Could you check a few things on this model? Use its own coordinates, in mm. A direction names the side the tool comes from. Give positions to 0.01 mm unless a question says otherwise; leave off trailing zeros. Loops run counter-clockwise (first coordinate to the right, second up) from the corner with the lowest first, then second, coordinate; pieces in that order, holes last. Notation, with made-up numbers: (-11, -17) -> (42, -17) arc R18 ccw to (42, -1) -> close; hole circle Ø2 at (79, 0.5). An arc over 180 degrees is marked (long way). Put each result on its own line as item: value.
```python
from build123d import *

# Parameters (mm, degrees)
F1_DEPTH = 63.5
F0_W     = 25.4
F0_H     = 19.05
F2_DEPTH = 25.4
F3_DEPTH = 7.9375


with BuildPart() as f1:
    # F0 (on Front) → F1 (new body, symmetric)
    with BuildSketch(Plane.XZ):
        Polygon((41.275, -9.525), (41.275, 9.525), (22.225, 9.525), (-41.275, 9.525), (-41.275, -9.525), align=None)
    extrude(amount=F1_DEPTH, both=True)

    # F0 (on Front) → F2 (join, symmetric)
    with BuildSketch(Plane.XZ):
        with BuildLine():
            Line((22.225, 9.525), (41.275, 9.525))
            Line((41.275, 9.525), (41.275, 27.0002))
            ThreePointArc((41.275, 27.0002), (45.9246798487, 38.2255201513), (57.15, 42.8752))
            Line((57.15, 42.8752), (60.325, 42.8752))
            Line((60.325, 42.8752), (60.325, 61.9252))
            Line((60.325, 61.9252), (57.15, 61.9252))
            ThreePointArc((57.15, 61.9252), (32.4542956671, 51.6959043329), (22.225, 27.0002))
            Line((22.225, 27.0002), (22.225, 9.525))
        make_face()
        with Locations((73.025, 52.4002)):
            Rectangle(F0_W, F0_H)
    extrude(amount=F2_DEPTH, both=True)

    # F0 (on Front) → F3 (join, symmetric)
    with BuildSketch(Plane.XZ):
        with BuildLine():
            Line((-41.275, 9.525), (22.225, 9.525))
            Line((22.225, 9.525), (22.225, 27.0002))
            ThreePointArc((22.225, 27.0002), (32.4542956671, 51.6959043329), (57.15, 61.9252))
            add(Edge.make_bspline(
                [(-41.275, 9.525), (-40.8389680088, 57.1731589735), (19.1717255543, 65.6824364242), (57.15, 61.9252)],
                knots=[0, 0, 0, 0, 111.5045361635, 111.5045361635, 111.5045361635, 111.5045361635], degree=3))
        make_face()
    extrude(amount=F3_DEPTH, both=True)


solid = f1.part
```
1. If we section it at B-B (z = -2.5): List the corners of the cut face in (x, y) for me (3 decimals), then the cut area to 3 significant figures.
Recorded:
outline: (-41.275, -63.5) -> (41.275, -63.5) -> (41.275, 63.5) -> (-41.275, 63.5) -> close
area: 10,500 mm^2
2. I need wall thicknesses on line 1 (Z direction, x = -9, y = 23) (3 decimals); line 2 (X direction, y = -17, z = 21.5) (3 decimals); line 3 (Z direction, x = 57, y = -14). Which ranges of each line are inside material? Lowest first, please.
Recorded:
line 1: z = -9.525 to 9.525
line 2: x = 22.225 to 41.275
line 3: z = 42.87 to 61.92
3. For faces 1 (the face through (72, 0, 61.925)), 2 (the face through (22.225, -17, 18)), 3 (the face through (71, 0, 42.875)), 4 (the face through (46, -25.4, 42)), which set-ups out of +Z, -Z, +X, -X, +Y, -Y let a thin tool reach every point of the face, with its end or its side?
Recorded:
face 1: +Z, +X, +Y, -Y
face 2: +Z, -X, -Y
face 3: -Z, +X, +Y, -Y
face 4: +Z, +X, -X, -Y
4. I'm going to push flat-ended pins straight in: pin 1 (14.5 mm diameter, centred on x = 71.5, y = -9.5, fed in from -Z); pin 2 (19 mm diameter, centred on y = 13, z = 20, fed in from -X); pin 3 (12 mm diameter, centred on x = 37, z = 27.5, fed in from +Y). Where does each tip first touch, or does it pass through?
Recorded:
pin 1: stops at z = 42.88
pin 2: stops at x = -41.2
pin 3: stops at y = 25.4
5. If we section it at C-C (x = 71.5): List the corners of the cut face in (y, z) for me.
Recorded:
outline: (-25.4, 42.88) -> (25.4, 42.88) -> (25.4, 61.93) -> (-25.4, 61.93) -> close
6. If we section it at A-A (y = -23.5): List the corners of the cut face in (x, z) for me (3 decimals).
Recorded:
outline: (-41.275, -9.525) -> (41.275, -9.525) -> (41.275, 27) arc R15.875 cw to (57.15, 42.875) -> (85.725, 42.875) -> (85.725, 61.925) -> (57.15, 61.925) arc R34.925 ccw to (22.225, 27) -> (22.225, 9.525) -> (-41.275, 9.525) -> close
